from build123d import *

# Parameters (mm, degrees)
SKETCH1_R           = 14.2875
SKETCH1_R_2         = 7.9375
SKETCH1_R_3         = 3.429
BOSS_EXTRUDE1_DEPTH = 3.175


with BuildPart() as part:
    # Sketch1 → Boss-Extrude1 (new body)
    with BuildSketch(Plane(origin=(0, 0, 0), x_dir=(0, 0, -1), z_dir=(1, 0, 0))):
        with BuildLine():
            Line((25.4, 57.15), (25.4, 28.398063314))
            ThreePointArc((25.4, 28.398063314), (24.8467304, 25.80568667), (23.283333333, 23.665052762))
            ThreePointArc((23.283333333, 23.665052762), (12.7, 0), (23.283333333, -23.665052762))
            ThreePointArc((23.283333333, -23.665052762), (24.8467304, -25.80568667), (25.4, -28.398063314))
            Line((25.4, -28.398063314), (25.4, -82.55))
            ThreePointArc((25.4, -82.55), (23.540128061, -87.040128061), (19.05, -88.9))
            Line((19.05, -88.9), (-1.575652176, -88.9))
            ThreePointArc((-1.575652176, -88.9), (-4.987504689, -87.905535681), (-7.330706623, -85.233625962))
            Line((-7.330706623, -85.233625962), (-16.304501832, -65.989260033))
            ThreePointArc((-16.304501832, -65.989260033), (-19.450268482, -62.883748133), (-23.860481018, -62.583619201))
            ThreePointArc((-23.860481018, -62.583619201), (-35.194449796, -57.475157953), (-31.822423449, -45.509178558))
            ThreePointArc((-31.822423449, -45.509178558), (-29.217505575, -41.937840594), (-29.574405884, -37.53185896))
            Line((-29.574405884, -37.53185896), (-42.070217791, -10.734503848))
            ThreePointArc((-42.070217791, -10.734503848), (-44.064116927, 4.410663713), (-37.010512242, 17.960512242))
            Line((-37.010512242, 17.960512242), (6.669103576, 61.640128061))
            ThreePointArc((6.669103576, 61.640128061), (8.729191841, 63.016635031), (11.159231637, 63.5))
            Line((11.159231637, 63.5), (19.05, 63.5))
            ThreePointArc((19.05, 63.5), (23.540128061, 61.640128061), (25.4, 57.15))
        make_face()
        with Locations((-19.05, 0)):
            Circle(SKETCH1_R, mode=Mode.SUBTRACT)
        with Locations((12.7, 38.1)):
            Circle(SKETCH1_R_2, mode=Mode.SUBTRACT)
        with Locations((12.7, -63.5)):
            Circle(SKETCH1_R_2, mode=Mode.SUBTRACT)
        with Locations((-26.561868124, -53.44971901)):
            Circle(SKETCH1_R_3, mode=Mode.SUBTRACT)
        with Locations((12.7, 53.975)):
            Circle(SKETCH1_R_3, mode=Mode.SUBTRACT)
        with Locations((-3.175, -63.5)):
            Circle(SKETCH1_R_3, mode=Mode.SUBTRACT)
        with Locations((12.7, -47.625)):
            Circle(SKETCH1_R_3, mode=Mode.SUBTRACT)
        with Locations((12.7, -79.375)):
            Circle(SKETCH1_R_3, mode=Mode.SUBTRACT)
        with Locations((-3.175, 38.1)):
            Circle(SKETCH1_R_3, mode=Mode.SUBTRACT)
        with Locations((12.7, 22.225)):
            Circle(SKETCH1_R_3, mode=Mode.SUBTRACT)
    extrude(amount=BOSS_EXTRUDE1_DEPTH)


solid = part.part
Geometry: final body of the model. Coordinates: model frame, mm. A direction names the side the tool comes from. Give positions to 0.01 mm unless a question says otherwise; leave off trailing zeros. Order: outer loops, then holes, each group sorted by start corner. A loop starts at its lowest first (then second) coordinate and runs counter-clockwise, first axis right, second up. Notation, with made-up numbers: (25.5, 42.5) -> (45.5, 42.5) arc R28 ccw to (45.5, 75.5) -> close; hole circle Ø4 at (-29.75, -29.75). An arc over 180 degrees is marked (long way). Put each result on its own line as item: value.
Q1. Section D-D, the plane x = 0.6. Count the separate pieces of the cut face and the enclosed holes in it, then the cut area to 3 significant figures.
Here are the results:
separate pieces: 1
enclosed holes: 10
area: 6,070 mm^2
Q2. Section A-A, the plane y = -3.5. Return loops of the section in (x, z) (1 decimal), then the cut area to 3 significant figures.
Here are the results:
outline: (0, -12.9) -> (3.2, -12.9) -> (3.2, 5.2) -> (0, 5.2) -> close; (0, 32.9) -> (3.2, 32.9) -> (3.2, 44.2) -> (0, 44.2) -> close
area: 93.3 mm^2
Q3. Section B-B, the plane z = 19.05. Return loops of the section in (x, y) (1 decimal), then the cut area to 3 significant figures.
Here are the results:
outline: (0, -63.1) -> (3.2, -63.1) -> (3.2, -14.3) -> (0, -14.3) -> close; (0, 14.3) -> (3.2, 14.3) -> (3.2, 35.9) -> (0, 35.9) -> close
area: 224 mm^2
Q4. Draft query along Z for faces 1 (the face through (1.57, 39.49, 15.48)), 2 (the face through (2, -55, -25.4)), 3 (the face through (1.565, 57.375, -12.254)). Return one class per face: released by +Z, released by -Z, zero draft, split by the parting line, or undercut.
Here are the results:
face 1: released by +Z
face 2: released by -Z
face 3: undercut
Q5. Pin query (flat end, axial travel): pin 1 (1.5 mm diameter, centred on x = 2, y = 8.5, fed in from -Z). Return the tip coordinate at first contact, or that it passes through.
Here are the results:
pin 1: stops at z = -14.08
Q6. Reachability of faces 4 (the face through (1.565, -24.321, 35.735)), 5 (the face through (1.57, -62.91, 19.39)), 6 (the face through (1.57, -25.77, -24.83)) from +Z, -Z, +X, -X, +Y, -Y: full face, straight path, thin tool, end or side. Return the list, or none.
Here are the results:
face 4: +Z, +X, -X
face 5: +X, -X, -Y
face 6: -Z, +X, -X
Q7. Section C-C, the plane y = 38.1. Return loops of the section in (x, z) (1 decimal).
Here are the results:
outline: (0, -25.4) -> (3.2, -25.4) -> (3.2, -20.6) -> (0, -20.6) -> close; (0, -4.8) -> (3.2, -4.8) -> (3.2, -0.3) -> (0, -0.3) -> close; (0, 6.6) -> (3.2, 6.6) -> (3.2, 16.9) -> (0, 16.9) -> close
Q8. Material intervals for L1, parallel to Z at x = 1.75, y = -64; L2, parallel to Y at x = 2.3, z = -7; L3, parallel to Y at x = 1.9, z = 24.5, sorted ascending.
Here are the results:
L1: z = -25.4 to -20.62, -4.78 to -0.22, 6.57 to 17.76
L2: y = -88.9 to -69.02, -57.98 to 32.58, 43.62 to 61.95
L3: y = -62.75 to -56.19, -50.71 to -13.21, 13.21 to 30.47
